CAD build for the part. Positions are in the model's coordinates, mm. Round coordinates to 2 decimals unless told otherwise and drop trailing zeros. Write each loop counter-clockwise with the first axis right and the second up, starting at its lowest first coordinate (ties: lowest second). Pieces come first, ordered by that corner, then holes. Notation, with made-up numbers: (22.25, -7) - (40.25, -7) arc R12 ccw to (40.25, 2) - close; hole circle Ø3 at (-16.5, 60). An arc over 180 degrees is marked (long way). Answer in a Markdown table with one row per item.
```python
from build123d import *

# Parameters (mm, degrees)
SKETCH1_R           = 1
BOSS_EXTRUDE1_DEPTH = 1.5


with BuildPart() as part:
    # Sketch1 → Boss-Extrude1 (new body)
    # profile 1 of 5: a face of its own
    with BuildSketch(Plane.XY):
        Polygon((0, 72), (-20, 72), (-35, 40), (-57.5, 40), (-57.5, 30), (-57.5, 20), (-35, 20), (-20, 0), (0, 0), (50, 0), (50, 25), (0, 25), align=None)
        with BuildLine():
            ThreePointArc((-40, 27.5), (-41.767766953, 28.232233047), (-42.5, 30))
            ThreePointArc((-42.5, 30), (-41.767766953, 31.767766953), (-40, 32.5))
            ThreePointArc((-40, 32.5), (-38.232233047, 31.767766953), (-37.5, 30))
            ThreePointArc((-37.5, 30), (-38.232233047, 28.232233047), (-40, 27.5))
        make_face(mode=Mode.SUBTRACT)
        with Locations((-15, 66.44)):
            Circle(SKETCH1_R, mode=Mode.SUBTRACT)
        with Locations((-5, 66.44)):
            Circle(SKETCH1_R, mode=Mode.SUBTRACT)
    # profile 2 of 5: a face of its own
    with BuildSketch(Plane.XY):
        with BuildLine():
            Line((-57.5, 30), (-57.5, 40))
            Line((-57.5, 40), (-75, 40))
            Line((-75, 40), (-75, 32.5))
            ThreePointArc((-75, 32.5), (-73.232233047, 31.767766953), (-72.5, 30))
            Line((-72.5, 30), (-57.5, 30))
        make_face()
    # profile 3 of 5: a face of its own
    with BuildSketch(Plane.XY):
        with BuildLine():
            Line((-57.5, 20), (-57.5, 30))
            Line((-57.5, 30), (-72.5, 30))
            ThreePointArc((-72.5, 30), (-73.232233047, 28.232233047), (-75, 27.5))
            Line((-75, 27.5), (-75, 20))
            Line((-75, 20), (-57.5, 20))
        make_face()
    # profile 4 of 5: a face of its own
    with BuildSketch(Plane.XY):
        with BuildLine():
            Line((-77.5, 30), (-80, 30))
            Line((-80, 30), (-80, 20))
            Line((-80, 20), (-75, 20))
            Line((-75, 20), (-75, 27.5))
            ThreePointArc((-75, 27.5), (-76.767766953, 28.232233047), (-77.5, 30))
        make_face()
    # profile 5 of 5: a face of its own
    with BuildSketch(Plane.XY):
        with BuildLine():
            Line((-75, 32.5), (-75, 40))
            Line((-75, 40), (-80, 40))
            Line((-80, 40), (-80, 30))
            Line((-80, 30), (-77.5, 30))
            ThreePointArc((-77.5, 30), (-76.767766953, 31.767766953), (-75, 32.5))
        make_face()
    extrude(amount=BOSS_EXTRUDE1_DEPTH)


solid = part.part
```
Q1. Saw through at A-A on z = 0.25. List the corners of the cut face in (x, y).
Computed:
| item | result |
|---|---|
| outline | (-80, 20) - (-35, 20) - (-20, 0) - (50, 0) - (50, 25) - (0, 25) - (0, 72) - (-20, 72) - (-35, 40) - (-80, 40) - close; hole circle Ø5 at (-75, 30); hole circle Ø5 at (-40, 30); hole circle Ø2 at (-15, 66.44); hole circle Ø2 at (-5, 66.44) |
Q2. Drill centre lines: line 1 (Y direction, x = -15, z = 0.3); line 2 (X direction, y = 66.44, z = 1.15); line 3 (Y direction, x = -56, z = 1.25). Where is each one in solid material? Low to high.
Computed:
| item | result |
|---|---|
| line 1 | y = 0 to 65.44, 67.44 to 72 |
| line 2 | x = -22.61 to -16, -14 to -6, -4 to 0 |
| line 3 | y = 20 to 40 |
Q3. Saw through at B-B on y = 35. List the corners of the cut face in (x, z).
Computed:
| item | result |
|---|---|
| outline | (-80, 0) - (0, 0) - (0, 1.5) - (-80, 1.5) - close |
Q4. Saw through at C-C on x = 24. List the corners of the cut face in (y, z).
Computed:
| item | result |
|---|---|
| outline | (0, 0) - (25, 0) - (25, 1.5) - (0, 1.5) - close |
Q5. Flat gauge pins, fed straight in: pin 1 (0.8 mm diameter, centred on x = 36.5, z = 0.5, fed in from +Y); pin 2 (1.6 mm diameter, centred on x = -5, y = 66.44, fed in from -Z) (3 decimals). Where does each tip first touch, or does it go through?
Computed:
| item | result |
|---|---|
| pin 1 | stops at y = 25 |
| pin 2 | passes through |
